```python
from build123d import *

# Parameters (mm, degrees)
F0_W     = 170
F0_H     = 210
F1_DEPTH = 300
F2_W     = 170
F2_H     = 65
F3_DEPTH = 1
F4_R     = 38.1
F4_R_2   = 5
F4_R_3   = 76.2
F5_DEPTH = 10


with BuildPart() as f1:
    # F0 (on Top) → F1 (new body)
    with BuildSketch(Plane.XY):
        Rectangle(F0_W, F0_H)
    extrude(amount=F1_DEPTH)

    # F2 (on face) → F3 (join)
    with BuildSketch(Plane(origin=(0, 105, 0), x_dir=(-1, 0, 0), z_dir=(0, 1, 0))):
        with Locations((0, 32.5)):
            Rectangle(F2_W, F2_H)
    extrude(amount=F3_DEPTH)

    # F4 (on face) → F5 (cut)
    with BuildSketch(Plane.XZ.offset(105)):
        with Locations((0, 237.059057)):
            Circle(F4_R)
        with Locations((0, 237.059057)):
            Circle(F4_R_2, mode=Mode.SUBTRACT)
        with Locations((0, 112.059531)):
            Circle(F4_R_3)
    extrude(amount=-F5_DEPTH, mode=Mode.SUBTRACT)


solid = f1.part
```
For this review, take the finished solid that the model builds, in its own axes (mm). A direction names the side the tool comes from. Round coordinates to 2 decimals unless told otherwise and drop trailing zeros. Loops run counter-clockwise (first coordinate to the right, second up) from the corner with the lowest first, then second, coordinate; pieces in that order, holes last.
(1) We need section D-D (z = 41). Give the boundary of the cut face in (x, y), plus the area to 3 significant figures.
Returned:
outline: (-85, -105) - (-27.51, -105) - (-27.51, -95) - (27.51, -95) - (27.51, -105) - (85, -105) - (85, 106) - (-85, 106) - close
area: 35,300 mm2
(2) Clearance check with flat-ended pins moving along their axes: P1, Ø3, axis at x = -39.5, z = 80, coming from the +Y side; P2, Ø3, axis at x = 22, z = 74, coming from the -Y side; P3, Ø0.5, axis at x = 22, y = 105.5, coming from the +Z side. State where each tip first meets the part, or that it passes through.
Returned:
P1: stops at y = 105
P2: stops at y = -95
P3: stops at z = 65
(3) We need section C-C (x = 48.5). Give the boundary of the cut face in (y, z), plus the area to 3 significant figures.
Returned:
outline: (-105, 0) - (106, 0) - (106, 65) - (105, 65) - (105, 300) - (-105, 300) - (-105, 170.83) - (-95, 170.83) - (-95, 53.29) - (-105, 53.29) - close
area: 61,900 mm2
(4) We need section B-B (z = 255.5). Give the boundary of the cut face in (x, y), plus the area to 3 significant figures.
Returned:
outline: (-85, -105) - (-33.34, -105) - (-33.34, -95) - (33.34, -95) - (33.34, -105) - (85, -105) - (85, 105) - (-85, 105) - close
area: 35,000 mm2
(5) Tool access review of faces 4 (the cylindrical face through (-1.084, -100.07, 232.178)), 5 (the flat face through (0, -105, 237)), 6 (the flat face through (-1, 105, 181)): name each direction out of +Z, -Z, +X, -X, +Y, -Y from which nothing blocks a thin tool from reaching the whole face with its end or side.
Returned:
face 4: -Y
face 5: +Z, -Z, +X, -X, -Y
face 6: +Z, +X, -X, +Y
(6) Mouldability with a two-part tool opening along X and no side actions: class faces 1 (the flat face through (-1, -95, 113)), 2 (the flat face through (85, -1, 148)), 3 (the flat face through (1, 106, 33)) as released by +X, released by -X, zero draft, split by the parting line, or undercut.
Returned:
face 1: undercut
face 2: released by +X
face 3: zero draft
(7) We need section A-A (x = 0). Give the boundary of the cut face in (y, z), plus the area to 3 significant figures.
Returned:
outline: (-105, 0) - (106, 0) - (106, 65) - (105, 65) - (105, 300) - (-105, 300) - (-105, 275.16) - (-95, 275.16) - (-95, 242.06) - (-105, 242.06) - (-105, 232.06) - (-95, 232.06) - (-95, 198.96) - (-105, 198.96) - (-105, 188.26) - (-95, 188.26) - (-95, 35.86) - (-105, 35.86) - close
area: 60,900 mm2
(8) Wall thickness on line 1 along Z through (x, y) = (0, -102.25); line 2 along Y through (x, z) = (6, 211.5); line 3 along Y through (x, z) = (-54, 276): over which ranges is each line inside the solid? List them lowest first.
Returned:
line 1: z = 0 to 35.86, 188.26 to 198.96, 232.06 to 242.06, 275.16 to 300
line 2: y = -95 to 105
line 3: y = -105 to 105
